Verification items for the finished model (mm, model axes). A direction names the side the tool comes from. Give positions to 0.01 mm unless a question says otherwise; leave off trailing zeros. Order: outer loops, then holes, each group sorted by start corner. A loop starts at its lowest first (then second) coordinate and runs counter-clockwise, first axis right, second up.
from build123d import *

# Parameters (mm, degrees)
KEYWAY_DEPTH               = 2.38125
HEXAGONAL_SKETCH_OUTSIDE_W = 58.716
HEXAGONAL_SKETCH_OUTSIDE_H = 58.716
HEXAGONAL_CUT_DEPTH        = 12.7


with BuildPart() as part:
    # Base Sketch → Base (revolve)
    with BuildSketch(Plane.XY, mode=Mode.PRIVATE) as base_sk:
        Polygon((0, 0), (152.4, 0), (152.4, 12.7), (146.05, 12.7), (146.05, 7.9375), (28.575, 7.9375), (28.575, 6.3373), (26.9748, 6.3373), (26.9748, 7.9502), (12.7, 7.9502), (12.7, 6.35), (0, 6.35), align=None)
    revolve(base_sk.sketch.rotate(Axis((-28.230722892, 0, 0), (1, 0, 0)), 90), axis=Axis((-28.230722892, 0, 0), (1, 0, 0)))

    # Keyway Sketch → Keyway (cut, symmetric)
    with BuildSketch(Plane.XY):
        with BuildLine():
            Line((69.85, 14.2875), (104.775, 14.2875))
            Line((104.775, 14.2875), (104.775, 8.7249))
            ThreePointArc((104.775, 8.7249), (103.84506403, 6.47983597), (101.6, 5.5499))
            Line((101.6, 5.5499), (73.025, 5.5499))
            ThreePointArc((73.025, 5.5499), (70.77993597, 6.47983597), (69.85, 8.7249))
            Line((69.85, 8.7249), (69.85, 14.2875))
        make_face()
    extrude(amount=KEYWAY_DEPTH, both=True, mode=Mode.SUBTRACT)

    # Hexagonal Sketch outside → Hexagonal Cut (cut)
    with BuildSketch(Plane.ZY):
        Rectangle(HEXAGONAL_SKETCH_OUTSIDE_W, HEXAGONAL_SKETCH_OUTSIDE_H)
        Polygon((3.175, 5.499261314), (-3.175, 5.499261314), (-6.35, 0), (-3.175, -5.499261314), (3.175, -5.499261314), (6.35, 0), align=None, mode=Mode.SUBTRACT)
    extrude(amount=-HEXAGONAL_CUT_DEPTH, mode=Mode.SUBTRACT)


solid = part.part
(1) Go/stop test with flat-tipped pins: pin 1 (8 mm diameter, centred on x = 43, z = 7.5, fed in from +Y); pin 2 (2 mm diameter, centred on x = 133, y = -9.5, fed in from -Z); pin 3 (0.6 mm diameter, centred on x = 85, y = 6.5, fed in from -Z); pin 4 (12 mm diameter, centred on x = 90, z = -8.5, fed in from +Y). Record where each tip stops, or that it passes through.
Solved:
pin 1: stops at y = 7.12
pin 2: passes through
pin 3: stops at z = -4.96
pin 4: stops at y = 7.53
(2) Scan lines: line 1 (X direction, y = 3.75, z = -5.25) (3 decimals); line 2 (X direction, y = 7, z = 2) (3 decimals); line 3 (X direction, y = 4.75, z = -10.75). Record each from-to range of solid material in increasing order.
Solved:
line 1: x = 12.7 to 26.975, 28.575 to 152.4
line 2: x = 12.7 to 26.975, 28.575 to 70.359, 104.266 to 152.4
line 3: x = 146.05 to 152.4
(3) Section check C-C, the plane x = 88.5. Enter the section's corners in (y, z) (1 decimal), then the cut area to 3 significant figures.
Solved:
outline: (5.5, -2.4) - (5.5, 2.4) - (7.6, 2.4) arc R7.9 ccw (long way) to (7.6, -2.4) - close
area: 187 mm2
(4) Section check D-D, the plane z = 10.5. Enter the section's corners in (x, y), then the cut area to 3 significant figures.
Solved:
outline: (146.05, -7.14) - (152.4, -7.14) - (152.4, 7.14) - (146.05, 7.14) - close
area: 90.7 mm2
(5) Section check B-B, the plane x = 30. Enter the section's corners in (y, z) (1 decimal).
Solved:
outline: circle Ø15.9 at (0, 0)
(6) Set-up check for faces 1 (the cylindrical face through (71.1, 6.2, 0)), 2 (the flat face through (6.261, -2.711, -4.785)), 3 (the flat face through (26.975, 6, 3)), 4 (the flat face through (146.05, 8.3, -0.2)): record each of +Z, -Z, +X, -X, +Y, -Y from which the full face is reachable in a straight line by a thin tool's end or side.
Solved:
face 1: +Y
face 2: -Z, -X, -Y
face 3: none
face 4: -X
